Geometry: see drawing. Coordinates: mm, zero at the bounding-box minimum. A direction names the side the tool comes from. Coordinates: 2 decimals unless noted, no trailing zeros. Loops run counter-clockwise (first coordinate to the right, second up) from the corner with the lowest first, then second, coordinate; pieces in that order, holes last. Notation, with made-up numbers: (84, -36.5) -> (110, -36.5) arc R8 cw to (110, -22.5) -> close; hole circle Ø9 at (69.25, -20). An arc over 180 degrees is marked (long way). One line per item, written item: value. Start each with the question number.
Item 1: Ray query, probe 1 along X at (y, z) = (0.65, 4); probe 2 along Z at (x, y) = (5.25, 0.85). Return the intervals inside material, ascending. Write a range as from..to.
Item 2: Section query C-C on y = 3. Return loops of the section in (x, z).
Item 3: Section query B-B on x = 4. Return loops of the section in (y, z), then the cut area to 3 significant figures.
Item 4: Mould query, pull axis Z, two halves, no side actions, for the marked faces 1, 2 and 3. Classes: +Z half, -Z half, draft (parallel to the pull), parting line (faces both ways), or undercut.
Item 5: Contact query for flat-ended pins moving along their axis: pin 1 Ø0.8 at (x, y) = (3, 4.5) entering from +Z; pin 2 Ø3 at (x, z) = (3, 4) entering from -Y; pin 3 Ø0.5 at (x, y) = (5.5, 4.5) entering from -Z. Output: stop coordinate, or through.
Item 6: Section query D-D on z = 5. Return loops of the section in (x, y).
Item 7: Section query A-A on z = 4. Return loops of the section in (x, y).
Item 8: Set-up query: the marked faces 4, 5 and 6. Return all of +Z, -Z, +X, -X, +Y, -Y with unobstructed straight access to the full face (end or side cutting, diameter ignored); none if empty.
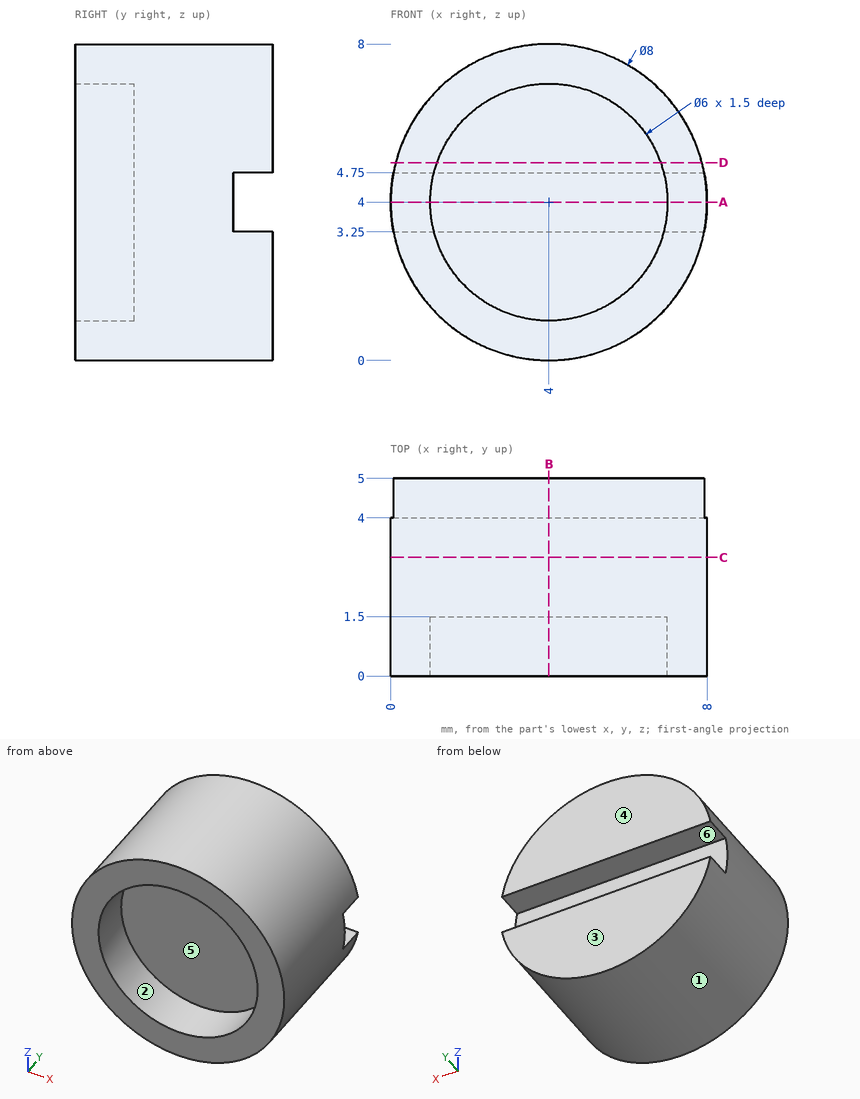
Reply:
1. probe 1: x = 0..1, 7..8
1. probe 2: z = 0.2..1.27, 6.73..7.8
2. outline: circle Ø8 at (4, 4)
3. outline: (0, 0) -> (5, 0) -> (5, 3.25) -> (4, 3.25) -> (4, 4.75) -> (5, 4.75) -> (5, 8) -> (0, 8) -> (0, 7) -> (1.5, 7) -> (1.5, 1) -> (0, 1) -> close
3. area: 29.5 mm²
4. face 1: parting line
4. face 2: undercut
4. face 3: draft
5. pin 1: stops at z = 7.95
5. pin 2: stops at y = 1.5
5. pin 3: stops at z = 0.2
6. outline: (0.13, 0) -> (1.17, 0) -> (1.17, 1.5) -> (6.83, 1.5) -> (6.83, 0) -> (7.87, 0) -> (7.87, 5) -> (0.13, 5) -> close
7. outline: (0, 0) -> (1, 0) -> (1, 1.5) -> (7, 1.5) -> (7, 0) -> (8, 0) -> (8, 4) -> (0, 4) -> close
8. face 4: +Z, -Z, +X, -X, +Y
8. face 5: -Y
8. face 6: +X, -X, +Y
